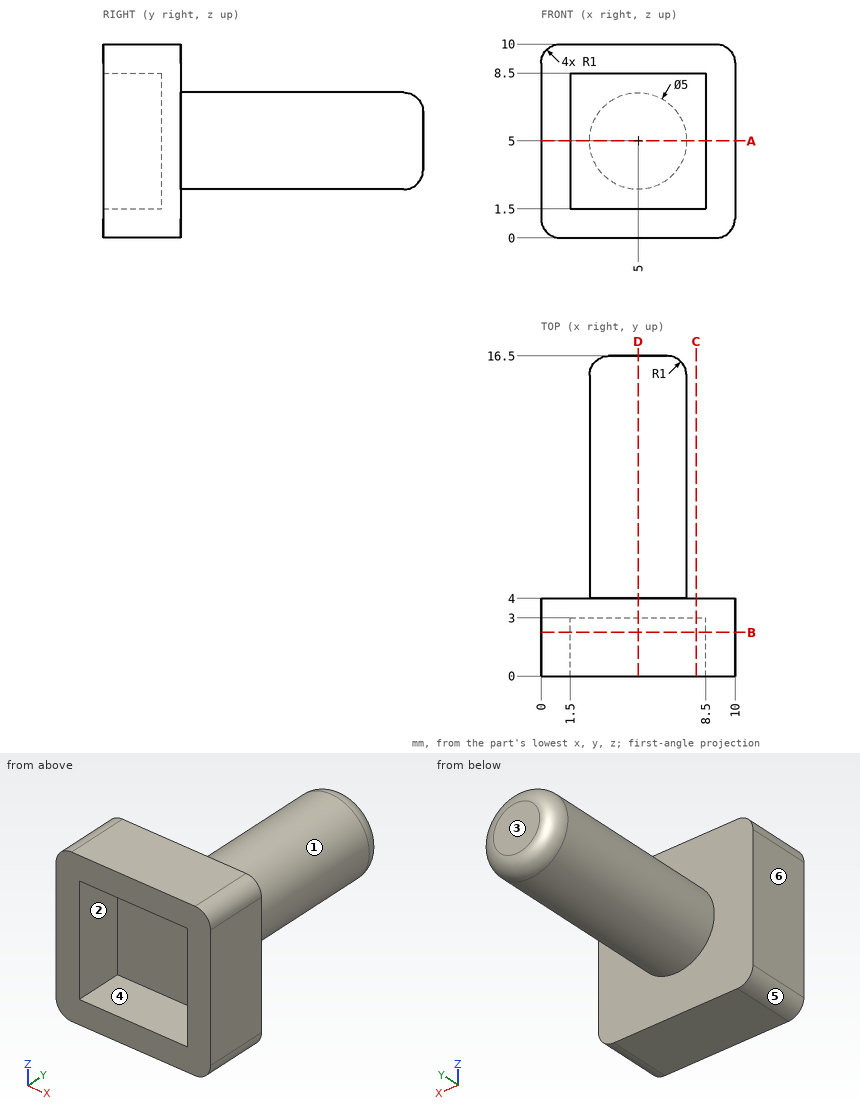
Design review of the part shown in the three views and the two pictorial views. Dimensions are in mm from the part's minimum x, y and z. A direction names the side the tool comes from. Coordinates: 2 decimals unless noted, no trailing zeros. Order: outer loops, then holes, each group sorted by start corner. A loop starts at its lowest first (then second) coordinate and runs counter-clockwise, first axis right, second up. Notation, with made-up numbers: (4.25, 50) - (36.25, 50) arc R26 cw to (36.25, 78) - close; hole circle Ø7 at (2, -6). An arc over 180 degrees is marked (long way). One line per question, with ' | ' between items.
Q1. Consider section B-B, the plane y = 2.25. Give the boundary of the cut face in (x, z), then the cut area to 3 significant figures.
Answer key:
outline: (0, 1) arc R1 ccw to (1, 0) - (9, 0) arc R1 ccw to (10, 1) - (10, 9) arc R1 ccw to (9, 10) - (1, 10) arc R1 ccw to (0, 9) - close; hole (1.5, 1.5) - (8.5, 1.5) - (8.5, 8.5) - (1.5, 8.5) - close | area: 50.1 mm2
Q2. Clearance check with flat-ended pins moving along their axes: pin 1 Ø3.5 at (x, z) = (6, 4.5) entering from -Y; pin 2 Ø1.5 at (x, y) = (4, 8.5) entering from -Z; pin 3 Ø3 at (x, y) = (8.5, 14.5) entering from -Z. State where each tip first meets the part, or that it passes through.
Answer key:
pin 1: stops at y = 3 | pin 2: stops at z = 2.51 | pin 3: stops at z = 3.5
Q3. The part is to be moulded in two halves that separate along Z. For the marked faces 4, 5 and 6, say which applies: +Z half, -Z half, draft (parallel to the pull), parting line (faces both ways), or undercut.
Answer key:
face 4: undercut | face 5: -Z half | face 6: draft
Q4. For the marked faces 1, 2 and 3, list the 3-axis set-ups (+Z, -Z, +X, -X, +Y, -Y) from which the entire face can be reached by the end or side of a thin tool; tool diameter is ignored.
Answer key:
face 1: +Y | face 2: -Y | face 3: +Z, -Z, +X, -X, +Y
Q5. Consider section D-D, the plane x = 5. Give the boundary of the cut face in (y, z).
Answer key:
outline: (0, 0) - (4, 0) - (4, 2.5) - (15.5, 2.5) arc R1 ccw to (16.5, 3.5) - (16.5, 6.5) arc R1 ccw to (15.5, 7.5) - (4, 7.5) - (4, 10) - (0, 10) - (0, 8.5) - (3, 8.5) - (3, 1.5) - (0, 1.5) - close
Q6. To check wall thickness, follow line 1 along X through (y, z) = (2, 1.75); line 2 along Y through (x, z) = (1.75, 1). State the ranges of each line that lie inside material, in increasing order.
Answer key:
line 1: x = 0 to 1.5, 8.5 to 10 | line 2: y = 0 to 4
Q7. Consider section C-C, the plane x = 8. Give the boundary of the cut face in (y, z).
Answer key:
outline: (0, 0) - (4, 0) - (4, 10) - (0, 10) - (0, 8.5) - (3, 8.5) - (3, 1.5) - (0, 1.5) - close
Q8. Consider section A-A, the plane z = 5. Give the boundary of the cut face in (x, y), then the cut area to 3 significant figures.
Answer key:
outline: (0, 0) - (1.5, 0) - (1.5, 3) - (8.5, 3) - (8.5, 0) - (10, 0) - (10, 4) - (7.5, 4) - (7.5, 15.5) arc R1 ccw to (6.5, 16.5) - (3.5, 16.5) arc R1 ccw to (2.5, 15.5) - (2.5, 4) - (0, 4) - close | area: 81.1 mm2
